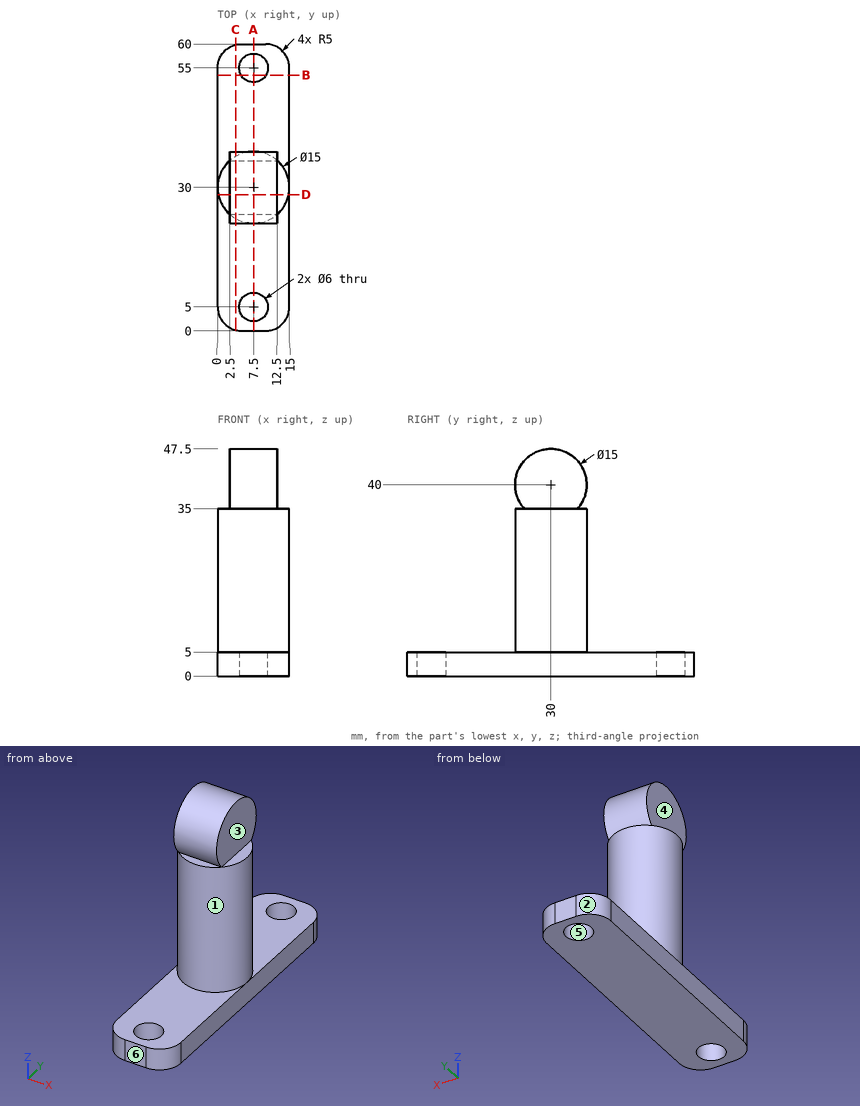
For this review, use the dimensioned drawing (mm, ordinates from the lowest corner) and the shaded views. A direction names the side the tool comes from. Coordinates: 2 decimals unless noted, no trailing zeros. Order: outer loops, then holes, each group sorted by start corner. A loop starts at its lowest first (then second) coordinate and runs counter-clockwise, first axis right, second up. Notation, with made-up numbers: (53, -27) -> (100, -27) arc R15 ccw to (100, -23) -> close; hole circle Ø9 at (-14.5, -18.5). An arc over 180 degrees is marked (long way). One line per item, written item: value. Start each with the question number.
Q1. Mouldability with a two-part tool opening along X and no side actions: class the marked faces 4, 5 and 6 as pulls with the +X half, pulls with the -X half, needs draft (parallel to the pull), parting line crosses it, or undercut.
Q2. For probe 1 along Y at (x, z) = (7.5, 2.7); probe 2 along X at (y, z) = (55, 2.55); probe 3 along Z at (x, y) = (4, 41.5), list the stretches that pass through material, from the lowest coordinate up.
Q3. Insertion check: pin 1 Ø0.8 at (x, y) = (14, 31) entering from +Z; pin 2 Ø3 at (x, z) = (7, 15.5) entering from +Y; pin 3 Ø8 at (x, z) = (4.5, 34) entering from -Y; pin 4 Ø5.5 at (x, y) = (7.5, 55) entering from -Z. Each pin has a flat end and moves straight along its axis. Give the tip position at first contact, or say it passes through.
Q4. Take a section at B-B, the plane y = 53.5. State the section outline as (x, z) points.
Q5. Tool access review of the marked faces 1, 2 and 3: name each direction out of +Z, -Z, +X, -X, +Y, -Y from which nothing blocks a thin tool from reaching the whole face with its end or side.
Q6. Take a section at D-D, the plane y = 28.5. State the section outline as (x, z) points.
Q7. Take a section at A-A, the plane x = 7.5. State the section outline as (y, z) points.
Q8. Take a section at C-C, the plane x = 3.75. State the section outline as (y, z) points, then the cut area to 3 significant figures.
Values follow:
1. face 4: pulls with the -X half
1. face 5: undercut
1. face 6: needs draft
2. probe 1: y = 0 to 2, 8 to 52, 58 to 60
2. probe 2: x = 0 to 4.5, 10.5 to 15
2. probe 3: z = 0 to 5
3. pin 1: stops at z = 35
3. pin 2: stops at y = 37.5
3. pin 3: stops at y = 22.5
3. pin 4: passes through
4. outline: (0, 0) -> (4.9, 0) -> (4.9, 5) -> (0, 5) -> close; (10.1, 0) -> (15, 0) -> (15, 5) -> (10.1, 5) -> close
5. face 1: none
5. face 2: +Z, -Z, -X, +Y
5. face 3: +Z, +X, +Y, -Y
6. outline: (0, 0) -> (15, 0) -> (15, 5) -> (14.85, 5) -> (14.85, 35) -> (12.5, 35) -> (12.5, 47.35) -> (2.5, 47.35) -> (2.5, 35) -> (0.15, 35) -> (0.15, 5) -> (0, 5) -> close
7. outline: (0, 0) -> (2, 0) -> (2, 5) -> (0, 5) -> close; (8, 0) -> (52, 0) -> (52, 5) -> (37.5, 5) -> (37.5, 35) -> (35.59, 35) arc R7.5 ccw (long way) to (24.41, 35) -> (22.5, 35) -> (22.5, 5) -> (8, 5) -> close; (58, 0) -> (60, 0) -> (60, 5) -> (58, 5) -> close
8. outline: (0.16, 0) -> (59.84, 0) -> (59.84, 5) -> (36.5, 5) -> (36.5, 35) -> (35.59, 35) arc R7.5 ccw (long way) to (24.41, 35) -> (23.5, 35) -> (23.5, 5) -> (0.16, 5) -> close
8. area: 845 mm2
